Can you work these out from the model? Positions are in its coordinate system, mm. A direction names the side the tool comes from. Round coordinates to 2 decimals unless told otherwise and drop trailing zeros. Order: outer loops, then holes, each group sorted by start corner. A loop starts at its lowest first (then second) coordinate and runs counter-clockwise, first axis right, second up. Notation, with made-up numbers: (64, 40) -> (110, 40) arc R21 cw to (110, 70) -> close; hole circle Ø8 at (-31, 27.5). An arc over 180 degrees is marked (long way). Use a Markdown table: item, result. Add a question column.
Q1. For faces 4 (the face through (1, -5, -2)), 5 (the face through (-2, -22.712, -5)), 6 (the face through (0, -23, -3)), which set-ups out of +Z, -Z, +X, -X, +Y, -Y let a thin tool reach every point of the face, with its end or its side?
Q2. We'd pull the mould along X, two halves only. Please class faces 1 (the face through (-3, -21, -1)), 2 (the face through (-10.421, -7, -5)), 3 (the face through (-2, 13.5, -4)): +X half, -X half, draft (parallel to the pull), parting line (faces both ways), or undercut.
Q3. If we section it at A-A on z = -5.25: List the corners of the cut face in (x, y) for me, plus the area to 3 significant figures.
Q4. If we section it at D-D on x = -6: List the corners of the cut face in (y, z) for me.
Q5. If we section it at B-B on y = -6: List the corners of the cut face in (x, z) for me.
Q6. I'm going to push flat-ended pins straight in: pin 1 Ø1.5 at (y, z) = (-11, -6) entering from -X; pin 2 Ø1.5 at (y, z) = (5, -2) entering from +X; pin 3 Ø3 at (x, z) = (10, -4) entering from -Y; pin 4 Ø17 at (x, y) = (-4, -13) entering from -Z. Where does each tip first touch, or does it pass through?
Q7. If we section it at C-C on z = -1.5: List the corners of the cut face in (x, y) for me, plus the area to 3 significant figures.
Q8. I need wall thicknesses on line 1 along X through (y, z) = (-10, -2.75); line 2 along Y through (x, z) = (17, -7.25); line 3 along Y through (x, z) = (-12, -1.5). Which ranges of each line are inside material? Lowest first, please. Write a range as [from, to].
```python
from build123d import *

# Parameters (mm, degrees)
SKETCH_1_W        = 4.436635541
SKETCH_1_H        = 2.8
EXTRUDE_1_DEPTH   = 8.8
SKETCH_1_W_2      = 7.689400099
SKETCH_1_H_2      = 13
EXTRUDE_1_2_DEPTH = 8.8
SKETCH_1_W_3      = 3
SKETCH_1_H_3      = 3.788471525
EXTRUDE_1_3_DEPTH = 8.8
EXTRUDE_1_4_DEPTH = 8.8
EXTRUDE_2_DEPTH   = 2


with BuildPart() as part:
    # Sketch 1 → Extrude 1 (new body)
    with BuildSketch(Plane.XY):
        with Locations((-12.63934737, -6.5)):
            Rectangle(SKETCH_1_W, SKETCH_1_H)
    extrude(amount=-EXTRUDE_1_DEPTH)


with BuildPart() as body_2:
    # Sketch 1 → Extrude 1 2 (new body)
    with BuildSketch(Plane.XY):
        with Locations((14.755299951, -6.5)):
            Rectangle(SKETCH_1_W_2, SKETCH_1_H_2)
    extrude(amount=-EXTRUDE_1_2_DEPTH)



with BuildPart() as body_3:
    # Sketch 1 → Extrude 1 3 (new body)
    with BuildSketch(Plane.XY):
        with Locations((-1.5, 11.605764238)):
            Rectangle(SKETCH_1_W_3, SKETCH_1_H_3)
    extrude(amount=-EXTRUDE_1_3_DEPTH)


with BuildPart() as body_4:
    # Sketch 1 → Extrude 1 4 (new body)
    with BuildSketch(Plane.XY):
        with Locations((-1.5, -24.605764238)):
            Rectangle(SKETCH_1_W_3, SKETCH_1_H_3)
    extrude(amount=-EXTRUDE_1_4_DEPTH)


with BuildPart() as body_2_1:
    add(body_2.part)

    add(body_3.part)  # Extrude 2 merges body 3

    add(body_4.part)  # Extrude 2 merges body 4
    # Sketch 2 → Extrude 2 (add)
    with BuildSketch(Plane.XY):
        Polygon((0, -13), (18.6, -13), (18.6, 0), (0, 0), (0, 13.5), (-3, 13.5), (-3, -5.1), (-14.85766514, -5.1), (-14.85766514, -7.9), (-3, -7.9), (-3, -26.5), (0, -26.5), align=None)
    extrude(amount=-EXTRUDE_2_DEPTH)


with BuildPart() as part_1:
    add(part.part)

    # Combine 1: union body 2
    add(body_2_1.part)


solid = part_1.part
```
Answer below:
| question | item | result |
|---|---|---|
| 1 | face 4 | -Z |
| 1 | face 5 | -Z, +X, -X |
| 1 | face 6 | +Z, -Z, +X, -Y |
| 2 | face 1 | -X half |
| 2 | face 2 | undercut |
| 2 | face 3 | draft |
| 3 | outline | (-14.86, -7.9) -> (-10.42, -7.9) -> (-10.42, -5.1) -> (-14.86, -5.1) -> close; (-3, -26.5) -> (0, -26.5) -> (0, -22.71) -> (-3, -22.71) -> close; (-3, 9.71) -> (0, 9.71) -> (0, 13.5) -> (-3, 13.5) -> close; (10.91, -13) -> (18.6, -13) -> (18.6, 0) -> (10.91, 0) -> close |
| 3 | area | 135 mm² |
| 4 | outline | (-7.9, -2) -> (-5.1, -2) -> (-5.1, 0) -> (-7.9, 0) -> close |
| 5 | outline | (-14.86, -8.8) -> (-10.42, -8.8) -> (-10.42, -2) -> (10.91, -2) -> (10.91, -8.8) -> (18.6, -8.8) -> (18.6, 0) -> (-14.86, 0) -> close |
| 6 | pin 1 | x = 10.91 |
| 6 | pin 2 | x = 0 |
| 6 | pin 3 | y = -13 |
| 6 | pin 4 | z = -8.8 |
| 7 | outline | (-14.86, -7.9) -> (-3, -7.9) -> (-3, -26.5) -> (0, -26.5) -> (0, -13) -> (18.6, -13) -> (18.6, 0) -> (0, 0) -> (0, 13.5) -> (-3, 13.5) -> (-3, -5.1) -> (-14.86, -5.1) -> close |
| 7 | area | 395 mm² |
| 8 | line 1 | [10.91, 18.6] |
| 8 | line 2 | [-13, 0] |
| 8 | line 3 | [-7.9, -5.1] |
